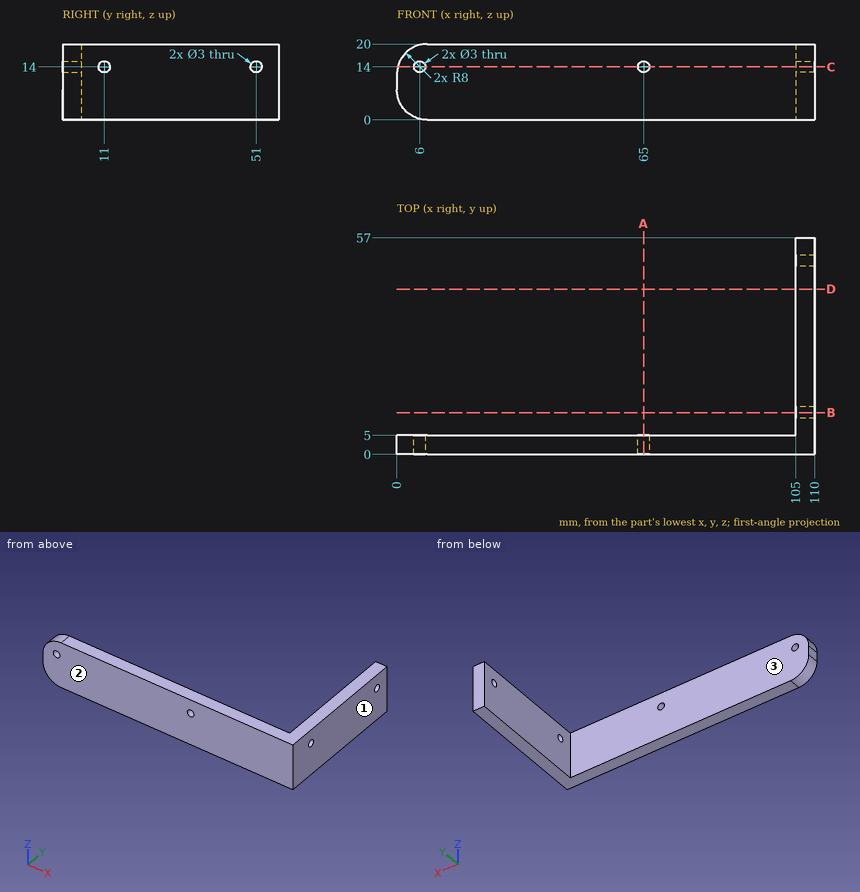
Check sheet for the drawn part. Datum: minimum x, y, z corner. Units: mm. Round coordinates to 2 decimals unless told otherwise and drop trailing zeros. Order: outer loops, then holes, each group sorted by start corner. A loop starts at its lowest first (then second) coordinate and runs counter-clockwise, first axis right, second up. Notation, with made-up numbers: (70.5, 49) -> (106.5, 49) arc R30 cw to (106.5, 86) -> close; hole circle Ø5 at (-33.5, 16.5). An arc over 180 degrees is marked (long way). Use CSV: the item, a comma, the result in double quotes.
(1) Draft check along Y on the marked faces 1, 2 and 3. Enter one of: pulls with the +Y half, pulls with the -Y half, needs draft (parallel to the pull), parting line crosses it, or undercut.
Worked out:
face 1,"needs draft"
face 2,"pulls with the -Y half"
face 3,"pulls with the +Y half"
(2) Cross-section at B-B (y = 11). Record the boundary of the cut face in (x, z), and give its area (3 significant figures).
Worked out:
outline,"(105, 0) -> (110, 0) -> (110, 12.5) -> (105, 12.5) -> close; (105, 15.5) -> (110, 15.5) -> (110, 20) -> (105, 20) -> close"
area,"85.0 mm²"
(3) Material ranges on line 1 along Y through (x, z) = (108.4, 14); line 2 along X through (y, z) = (2.1, 14); line 3 along Z through (x, y) = (65, 1), recorded low to high. Write a range as from..to.
Worked out:
line 1,"0..9.5, 12.5..49.5, 52.5..57"
line 2,"0.25..4.5, 7.5..63.5, 66.5..110"
line 3,"0..12.5, 15.5..20"
(4) Depth check by flat-ended pin: pin 1 (6 mm diameter, centred on x = 80, z = 16, fed in from -Y); pin 2 (6 mm diameter, centred on y = 46.5, z = 8, fed in from -X); pin 3 (2.5 mm diameter, centred on x = 65, z = 14, fed in from -Y); pin 4 (10 mm diameter, centred on x = 67.5, z = 5.5, fed in from +Y). Enter the tip coordinate at first touch or a pass-through.
Worked out:
pin 1,"y = 0"
pin 2,"x = 105"
pin 3,"through"
pin 4,"y = 5"
(5) Cross-section at C-C (z = 14). Record the boundary of the cut face in (x, y), and give its area (3 significant figures).
Worked out:
outline,"(0.25, 0) -> (4.5, 0) -> (4.5, 5) -> (0.25, 5) -> close; (7.5, 0) -> (63.5, 0) -> (63.5, 5) -> (7.5, 5) -> close; (66.5, 0) -> (110, 0) -> (110, 9.5) -> (105, 9.5) -> (105, 5) -> (66.5, 5) -> close; (105, 12.5) -> (110, 12.5) -> (110, 49.5) -> (105, 49.5) -> close; (105, 52.5) -> (110, 52.5) -> (110, 57) -> (105, 57) -> close"
area,"749 mm²"
(6) Cross-section at A-A (x = 65). Record the boundary of the cut face in (y, z), and give its area (3 significant figures).
Worked out:
outline,"(0, 0) -> (5, 0) -> (5, 12.5) -> (0, 12.5) -> close; (0, 15.5) -> (5, 15.5) -> (5, 20) -> (0, 20) -> close"
area,"85.0 mm²"
(7) Cross-section at D-D (y = 43.5). Record the boundary of the cut face in (x, z).
Worked out:
outline,"(105, 0) -> (110, 0) -> (110, 20) -> (105, 20) -> close"
